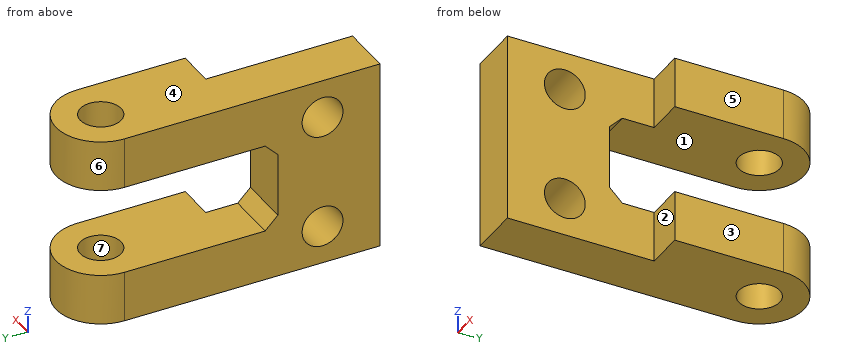
from build123d import *

# Parameters (mm, degrees)
SKETCH_1_R          = 1.6
EXTRUDE_1_DEPTH     = 15
SKETCH_3_W          = 7
SKETCH_3_H          = 18.899287815
CUT_EXTRUDE_2_DEPTH = 26.961509971
SKETCH_4_W          = 3
SKETCH_4_H          = 17
CUT_EXTRUDE_3_DEPTH = 26.243811123
SKETCH_5_R          = 1.6
CUT_EXTRUDE_4_DEPTH = 10
CHAMFER_1_SIZE      = 1


with BuildPart() as part:
    # 草图1 → 凸台-拉伸1 (new body)
    with BuildSketch(Plane.XY):
        with BuildLine():
            Line((-3.5, -20), (-3.5, 0))
            ThreePointArc((-3.5, 0), (0, 3.5), (3.5, 0))
            Line((3.5, 0), (3.5, -20))
            Line((3.5, -20), (-3.5, -20))
        make_face()
        Circle(SKETCH_1_R, mode=Mode.SUBTRACT)
    extrude(amount=EXTRUDE_1_DEPTH)

    # 草图3 → 切除-拉伸2 (cut, through all)
    with BuildSketch(Plane.ZY.offset(3.5)):
        with Locations((7.5, -2.550356092)):
            Rectangle(SKETCH_3_W, SKETCH_3_H)
    extrude(amount=-CUT_EXTRUDE_2_DEPTH, mode=Mode.SUBTRACT)

    # 草图4 → 切除-拉伸3 (cut, through all)
    with BuildSketch(Plane(origin=(0, 0, 0), x_dir=(-1, 0, 0), z_dir=(0, 0, -1))):
        with Locations((-2, -17)):
            Rectangle(SKETCH_4_W, SKETCH_4_H)
    extrude(amount=-CUT_EXTRUDE_3_DEPTH, mode=Mode.SUBTRACT)

    # 草图5 → 切除-拉伸4 (cut)
    with BuildSketch(Plane.ZY.offset(3.5)):
        with Locations(Location((12, -15.5, 0), (0, 0, 270))):
            Circle(SKETCH_5_R)
        with Locations(Location((3, -15.5, 0), (0, 0, 270))):
            Circle(SKETCH_5_R)
    extrude(amount=-CUT_EXTRUDE_4_DEPTH, mode=Mode.SUBTRACT)

    # 倒角1
    chamfer_1_edges = [part.edges().sort_by_distance(p)[0] for p in [
        (-1.5, -12, 11),
        (-1.5, -12, 4),
    ]]
    chamfer(chamfer_1_edges, length=CHAMFER_1_SIZE)


solid = part.part
Read the model definition and answer for the solid it produces. Units are mm, in the model's axes. Face numbers are marked on the shaded views. A direction names the side the tool comes from. Round coordinates to 2 decimals unless told otherwise and drop trailing zeros. Loops run counter-clockwise (first coordinate to the right, second up) from the corner with the lowest first, then second, coordinate; pieces in that order, holes last. Notation, with made-up numbers: (4.5, 32) - (26.5, 32) arc R18 ccw to (26.5, 38) - close; hole circle Ø1 at (8.5, -19). An arc over 180 degrees is marked (long way). One line per question, with ' | ' between items. Start each with the question number.
Q1. Flat-ended cylindrical pins translate along their axes: pin 1 (1.5 mm diameter, centred on x = 1.5, z = 2.5, fed in from -Y); pin 2 (3 mm diameter, centred on x = 0, z = 8, fed in from +Y). Find the tip coordinate at first contact, or state that the pin passes through.
Q2. Section C-C on y = -15.5 is taken. Give the vertices of the cut face in (x, z), plus the area to 3 significant figures.
Q3. Find the intervals of material crossed by L1, parallel to Z at x = -0.95, y = -15.5; L2, parallel to X at y = 0, z = 13.95; L3, parallel to Z at x = -2, y = -3.5, in increasing order.
Q4. Section B-B on z = 12 is taken. Give the vertices of the cut face in (x, y).
Q5. For the marked faces 1, 2 and 3, determine the directions among +Z, -Z, +X, -X, +Y, -Y from which every point of the face is accessible in a straight line to the end or side of a thin tool.
Q6. Section A-A on x = 0 is taken. Give the vertices of the cut face in (y, z), plus the area to 3 significant figures.
Q7. Section D-D on y = -2.25 is taken. Give the vertices of the cut face in (x, z).
Q8. For a pull along X with two mould halves and no side action, classify the marked faces 4, 5, 6 and 7 as +X half, -X half, draft (parallel to the pull), parting line (faces both ways), or undercut.
Established:
1) pin 1: y = -8.5 | pin 2: y = -12
2) outline: (-3.5, 0) - (0.5, 0) - (0.5, 1.4) - (-3.5, 1.4) - close; (-3.5, 4.6) - (0.5, 4.6) - (0.5, 10.4) - (-3.5, 10.4) - close; (-3.5, 13.6) - (0.5, 13.6) - (0.5, 15) - (-3.5, 15) - close | area: 34.4 mm²
3) L1: 0 to 1.4, 4.6 to 10.4, 13.6 to 15 | L2: -3.5 to -1.6, 1.6 to 3.5 | L3: 0 to 4, 11 to 15
4) outline: (-3.5, -20) - (0.5, -20) - (0.5, -17.1) - (-3.5, -17.1) - close; (-3.5, -13.9) - (0.5, -13.9) - (0.5, -8.5) - (3.5, -8.5) - (3.5, 0) arc R3.5 ccw to (-3.5, 0) - close; hole circle Ø3.2 at (0, 0)
5) face 1: +X, -X, +Y | face 2: +Z, -Z, +X, -Y | face 3: +Z, -Z, +X, +Y, -Y
6) outline: (-20, 0) - (-1.6, 0) - (-1.6, 4) - (-11, 4) - (-12, 5) - (-12, 10) - (-11, 11) - (-1.6, 11) - (-1.6, 15) - (-20, 15) - close; (1.6, 0) - (3.5, 0) - (3.5, 4) - (1.6, 4) - close; (1.6, 11) - (3.5, 11) - (3.5, 15) - (1.6, 15) - close; hole circle Ø3.2 at (-15.5, 3); hole circle Ø3.2 at (-15.5, 12) | area: 203 mm²
7) outline: (-3.5, 0) - (3.5, 0) - (3.5, 4) - (-3.5, 4) - close; (-3.5, 11) - (3.5, 11) - (3.5, 15) - (-3.5, 15) - close
8) face 4: draft | face 5: +X half | face 6: parting line | face 7: undercut
